Input: dimensioned drawing with shaded views. Units: mm. Origin: part minimum x, y, z. Round coordinates to 2 decimals unless told otherwise and drop trailing zeros. Loops run counter-clockwise (first coordinate to the right, second up) from the corner with the lowest first, then second, coordinate; pieces in that order, holes last. Notation, with made-up numbers: M -20.75,27.5 L -0.75,27.5 A5 ccw -0.75,31.5 Z; hole C 28.25,58 d8. An arc over 180 degrees is marked long. One line per item, written item: value.
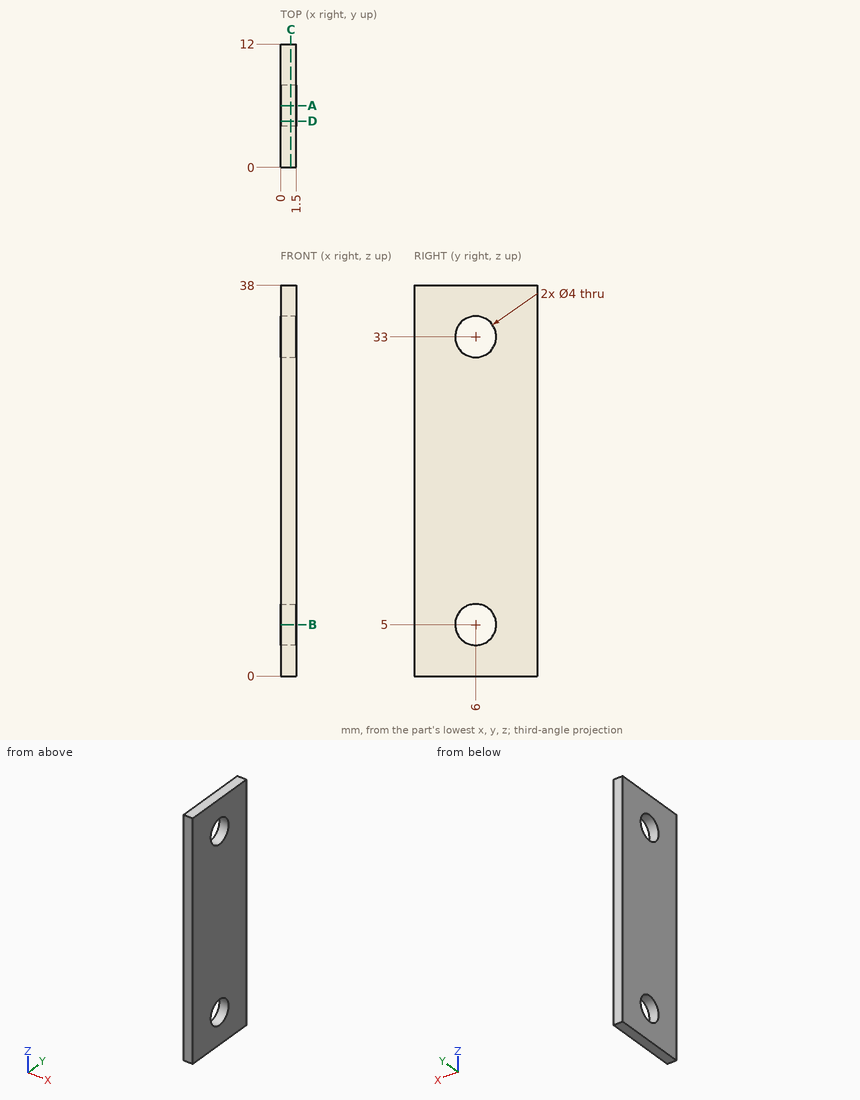
1. Section query A-A (y = 6). Return the cut outline in (x, z), and give its area (3 significant figures).
Report:
outline: M 0,0 L 1.5,0 L 1.5,3 L 0,3 Z; M 0,7 L 1.5,7 L 1.5,31 L 0,31 Z; M 0,35 L 1.5,35 L 1.5,38 L 0,38 Z
area: 45.0 mm2
2. Section query B-B (z = 5). Return the cut outline in (x, y).
Report:
outline: M 0,0 L 1.5,0 L 1.5,4 L 0,4 Z; M 0,8 L 1.5,8 L 1.5,12 L 0,12 Z
3. Ray query, line 1 (Y direction, x = 1, z = 33); line 2 (Y direction, x = 0.35, z = 32). Return the intervals inside material, ascending. Write a range as [from, to].
Report:
line 1: y = [0, 4], [8, 12]
line 2: y = [0, 4.27], [7.73, 12]
4. Section query D-D (y = 4.5). Return the cut outline in (x, z).
Report:
outline: M 0,0 L 1.5,0 L 1.5,3.68 L 0,3.68 Z; M 0,6.32 L 1.5,6.32 L 1.5,31.68 L 0,31.68 Z; M 0,34.32 L 1.5,34.32 L 1.5,38 L 0,38 Z
5. Section query C-C (x = 1). Return the cut outline in (y, z).
Report:
outline: M 0,0 L 12,0 L 12,38 L 0,38 Z; hole C 6,5 d4; hole C 6,33 d4
